Geometry: see drawing. Coordinates: mm, zero at the bounding-box minimum. A direction names the side the tool comes from. Coordinates: 2 decimals unless noted, no trailing zeros. Loops run counter-clockwise (first coordinate to the right, second up) from the corner with the lowest first, then second, coordinate; pieces in that order, holes last. Notation, with made-up numbers: M 26,-27 L 45,-27 A27 ccw 45,10 Z; hole C 6.5,57.25 d4. An arc over 180 degrees is marked long. One line per question, with ' | ' between items. Start each with the question number.
1. Section query C-C, the plane z = 21.5. Output: boundary loops of the cut face in (x, y) (1 decimal).
2. Section query A-A, the plane z = 35. Output: boundary loops of the cut face in (x, y) (1 decimal).
3. Section query D-D, the plane x = 24. Output: boundary loops of the cut face in (y, z).
4. Pin query (flat end, axial travel): P1, Ø5.5, axis at x = 33.5, z = 21.5, coming from the +Y side; P2, Ø8, axis at y = 85.5, z = 33, coming from the +X side; P3, Ø1, axis at y = 69, z = 41.5, coming from the -X side; P4, Ø15, axis at x = 17.78, y = 17.72, coming from the +Z side. Return the tip coordinate at first contact, or that it passes through.
5. Section query B-B, the plane x = 17.78. State how many separate pieces and enclosed holes the cut face has, and give its area (3 significant figures).
6. Mould query, pull axis Z, two halves, no side actions, for the marked faces 1, 2, 3 and 4. Classes: pulls with the +Z half, pulls with the -Z half, needs draft (parallel to the pull), parting line crosses it, or undercut.
7. Access query for the marked faces 5, 6, 7 and 8. Directions: +Z, -Z, +X, -X, +Y, -Y. A direction counts if a zero-diameter tool reaches every point of the face in a straight line with its end or side. Return the directions, or none.
8. Ray query, probe 1 along Y at (x, z) = (17.78, 33.5) (1 decimal); probe 2 along Y at (x, z) = (20.5, 20.5) (1 decimal); probe 3 along Y at (x, z) = (12.25, 24.13). Return the intervals inside material, ascending.
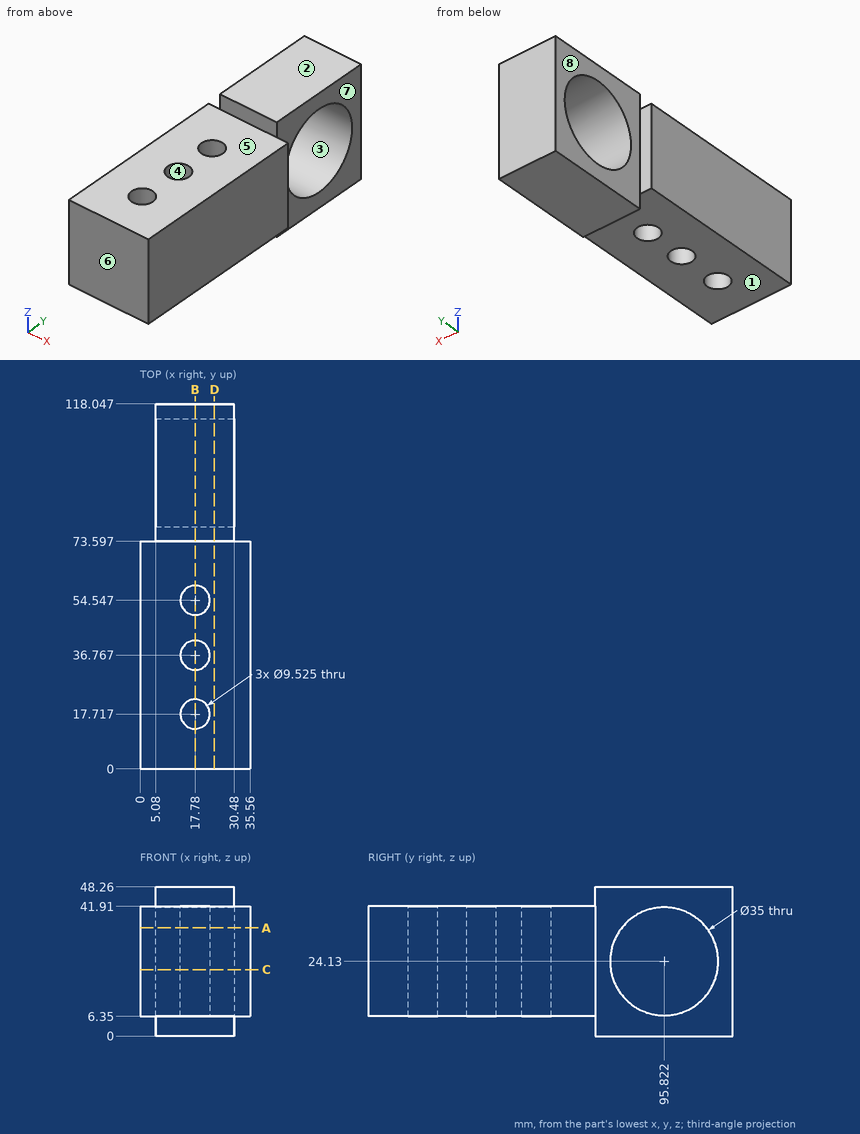
Taken from the geometry:
1) outline: M 0,0 L 35.6,0 L 35.6,73.6 L 30.5,73.6 L 30.5,78.5 L 5.1,78.5 L 5.1,73.6 L 0,73.6 Z; M 5.1,113.1 L 30.5,113.1 L 30.5,118 L 5.1,118 Z; hole C 17.8,17.7 d9.5; hole C 17.8,36.8 d9.5; hole C 17.8,54.5 d9.5
2) outline: M 0,0 L 35.6,0 L 35.6,73.6 L 30.5,73.6 L 30.5,82.1 L 5.1,82.1 L 5.1,73.6 L 0,73.6 Z; M 5.1,109.5 L 30.5,109.5 L 30.5,118 L 5.1,118 Z; hole C 17.8,17.7 d9.5; hole C 17.8,36.8 d9.5; hole C 17.8,54.5 d9.5
3) outline: M 0,6.35 L 73.6,6.35 L 73.6,0 L 118.05,0 L 118.05,48.26 L 73.6,48.26 L 73.6,41.91 L 0,41.91 Z; hole C 95.82,24.13 d35
4) P1: y = 73.6 | P2: x = 30.48 | P3: x = 0 | P4: z = 41.91
5) separate pieces: 4 | enclosed holes: 1 | area: 2,780 mm^2
6) face 1: pulls with the -Z half | face 2: pulls with the +Z half | face 3: undercut | face 4: needs draft
7) face 5: +Z, +X, -X, -Y | face 6: +Z, -Z, +X, -X, -Y | face 7: +Z, -Z, +X, +Y | face 8: +Z, -Z, -X, +Y
8) probe 1: 0 to 13, 22.5 to 32, 41.5 to 49.8, 59.3 to 81, 110.6 to 118 | probe 2: 0 to 13.8, 21.6 to 32.9, 40.7 to 50.6, 58.5 to 78.7, 112.9 to 118 | probe 3: 0 to 78.32, 113.32 to 118.05
